Can you work these out from the model? Positions are in its coordinate system, mm. Face numbers are marked on the shaded views. A direction names the side the tool comes from. Give positions to 0.01 mm unless a question says otherwise; leave off trailing zeros. Return JSON: item names as keys, results as strings. Group by question number.
Q1. Will these pins go through, and if not, where does the flat tip stop? pin 1 (5 mm diameter, centred on x = -35.5, y = -1117.5, fed in from +Z); pin 2 (5 mm diameter, centred on y = -1086.5, z = 99.5, fed in from +X); pin 3 (8 mm diameter, centred on x = -77, y = -1055, fed in from -Z).
Q2. Thinking about a two-plate mould opening in Y: for the marked faces 3, 4 and 5, which applies, pulls with the +Y half, pulls with the -Y half, needs draft (parallel to the pull), parting line crosses it, or undercut?
Q3. I need wall thicknesses on line 1 along Y through (x, z) = (-16.5, -124); line 2 along Z through (x, y) = (-14.5, -901.5); line 3 along Z through (x, y) = (-75.5, -909.5). Which ranges of each line are inside material? Lowest first, please. Write a range as [from, to].
Q4. Which directions (+Z, -Z, +X, -X, +Y, -Y) give clear straight access to the entire face, cutting with the end or side of a thin tool? Please do the marked faces 1 and 2.
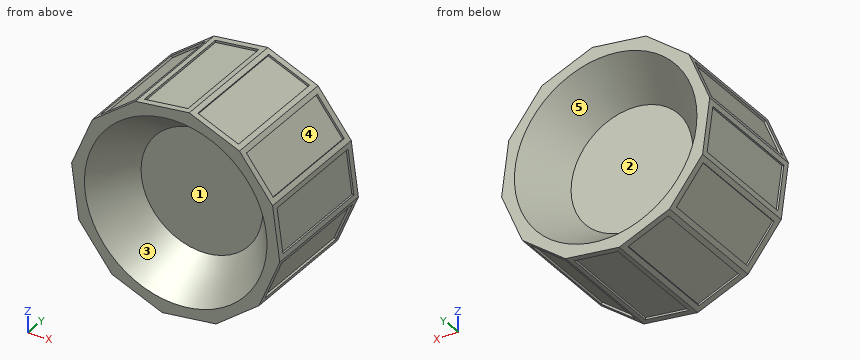
```python
from build123d import *

# Parameters (mm, degrees)
SKETCH_1_R               = 90
SKETCH_1_R_2             = 50
EXTRUDE_1_DEPTH          = 50
SKETCH_5_R               = 150
EXTRUDE_2_DEPTH          = 100
SKETCH_6_R               = 150
SKETCH_8_R               = 225
CUT_EXTRUDE_1_DEPTH      = 5
PATTERN_CIRCULAR_1_COUNT = 12


with BuildPart() as part:
    # 草图1 → 凸台-拉伸1 (new, symmetric)
    with BuildSketch(Plane(origin=(0, -1025, 0), x_dir=(-1, 0, 0), z_dir=(0, 1, 0))):
        with Locations(Location((0, 0, 0), (0, 0, 90))):
            Circle(SKETCH_1_R)
        with Locations(Location((0, 0, 0), (0, 0, 90))):
            Circle(SKETCH_1_R_2, mode=Mode.SUBTRACT)
    extrude(amount=EXTRUDE_1_DEPTH, both=True)

    # 草图5 → 凸台-拉伸2 (add)
    with BuildSketch(Plane(origin=(0, -975, 0), x_dir=(-1, 0, 0), z_dir=(0, 1, 0))):
        with Locations(Location((0, 0, 0), (0, 0, 90))):
            Circle(SKETCH_5_R)
    extrude(amount=-EXTRUDE_2_DEPTH)

    # 凸台-拉伸4: read off the stored shape, not the designer's step
    # 凸台-拉伸4: loft between two sections, ruled curve by curve
    extrude_4_from = [
        Edge.make_line((-33.353210676, -1175, -256.660985437), (-157.215220461, -1175, -205.598328211)),
        Edge.make_line((-157.215220461, -1175, -205.598328211), (-238.951538886, -1175, -99.445764975)),
        Edge.make_line((-238.951538886, -1175, -99.445764975), (-256.660985437, -1175, 33.353210676)),
        Edge.make_line((-256.660985437, -1175, 33.353210676), (-205.598328211, -1175, 157.215220461)),
        Edge.make_line((-205.598328211, -1175, 157.215220461), (-99.445764975, -1175, 238.951538886)),
        Edge.make_line((-99.445764975, -1175, 238.951538886), (33.353210676, -1175, 256.660985437)),
        Edge.make_line((33.353210676, -1175, 256.660985437), (157.215220461, -1175, 205.598328211)),
        Edge.make_line((157.215220461, -1175, 205.598328211), (238.951538886, -1175, 99.445764975)),
        Edge.make_line((238.951538886, -1175, 99.445764975), (256.660985437, -1175, -33.353210676)),
        Edge.make_line((256.660985437, -1175, -33.353210676), (205.598328211, -1175, -157.215220461)),
        Edge.make_line((205.598328211, -1175, -157.215220461), (99.445764975, -1175, -238.951538886)),
        Edge.make_line((99.445764975, -1175, -238.951538886), (-33.353210676, -1175, -256.660985437)),
    ]
    extrude_4_to = [
        Edge.make_line((-33.353210676, -875, -256.660985437), (-157.215220461, -875, -205.598328211)),
        Edge.make_line((-157.215220461, -875, -205.598328211), (-238.951538886, -875, -99.445764975)),
        Edge.make_line((-238.951538886, -875, -99.445764975), (-256.660985437, -875, 33.353210676)),
        Edge.make_line((-256.660985437, -875, 33.353210676), (-205.598328211, -875, 157.215220461)),
        Edge.make_line((-205.598328211, -875, 157.215220461), (-99.445764975, -875, 238.951538886)),
        Edge.make_line((-99.445764975, -875, 238.951538886), (33.353210676, -875, 256.660985437)),
        Edge.make_line((33.353210676, -875, 256.660985437), (157.215220461, -875, 205.598328211)),
        Edge.make_line((157.215220461, -875, 205.598328211), (238.951538886, -875, 99.445764975)),
        Edge.make_line((238.951538886, -875, 99.445764975), (256.660985437, -875, -33.353210676)),
        Edge.make_line((256.660985437, -875, -33.353210676), (205.598328211, -875, -157.215220461)),
        Edge.make_line((205.598328211, -875, -157.215220461), (99.445764975, -875, -238.951538886)),
        Edge.make_line((99.445764975, -875, -238.951538886), (-33.353210676, -875, -256.660985437)),
    ]
    extrude_4 = Solid(Shell([*[Face.make_surface_from_curves(extrude_4_from[k], extrude_4_to[k]) for k in range(12)], Face(Wire(extrude_4_from)), Face(Wire(extrude_4_to))]))
    add(extrude_4)

    # 草图6 → 切除-放样3 section 0
    with BuildSketch(Plane(origin=(0, -1075, 0), x_dir=(-1, 0, 0), z_dir=(0, 1, 0))):
        Circle(SKETCH_6_R)
    # 草图8 → 切除-放样3 section 1
    with BuildSketch(Plane(origin=(0, -1175, 0), x_dir=(-1, 0, 0), z_dir=(0, 1, 0))):
        Circle(SKETCH_8_R)
    loft_3 = loft(mode=Mode.SUBTRACT)

    # 镜向2: 切除-放样3 across plane
    add(loft_3.mirror(Plane.ZX.offset(-1025)), mode=Mode.SUBTRACT)

    # 草图9 → 切除-拉伸1 (cut)
    with BuildSketch(Plane(origin=(231.129656824, 0, -95.284215569), x_dir=(-0.3811368622740284, 0, -0.9245186272952581), z_dir=(0.9245186272952581, 0, -0.3811368622740284))):
        Polygon((-54.297116462, -889.659578346), (-54.297116462, -1146.583758404), (54.297116462, -903.416241596), (54.297116462, -889.659578346), align=None)
        Polygon((54.297116462, -903.416241596), (-54.297116462, -1146.583758404), (-54.297116462, -1160.340421654), (54.297116462, -1160.340421654), align=None)
    cut_extrude_1 = extrude(amount=-CUT_EXTRUDE_1_DEPTH, mode=Mode.SUBTRACT)

    # 阵列(圆周)1: 切除-拉伸1 ×12 about axis
    pattern_circular_1_axis = Axis((0, 0, 0), (0, 1, 0))
    for i in range(1, PATTERN_CIRCULAR_1_COUNT):
        add(cut_extrude_1.rotate(pattern_circular_1_axis, i * 360 / PATTERN_CIRCULAR_1_COUNT), mode=Mode.SUBTRACT)


solid = part.part
```
Ans:
{
 "1": {"pin 1": "stops at z = 242.77", "pin 2": "stops at x = 239.28", "pin 3": "stops at z = -234.91"},
 "2": {"face 3": "pulls with the -Y half", "face 4": "undercut", "face 5": "pulls with the +Y half"},
 "3": {"line 1": "y = [-1075, -975]", "line 2": "z = [-249.1, -204.61], [204.61, 245.24]", "line 3": "z = [-233.88, -184.26], [184.26, 237.1]"},
 "4": {"face 1": "-Y", "face 2": "+Y"}
}
